from build123d import *

# Parameters (mm, degrees)
PRISM070_DEPTH                = 10
PRISM070_PITCH_ANGLE          = 90
PRISM071_DEPTH                = 10
PRISM071_PITCH_ANGLE          = 90
PRISM072_DEPTH                = 10
PRISM072_PITCH_ANGLE          = 90
PRISM073_DEPTH                = 10
PRISM073_PITCH_ANGLE          = 90
CUBE082_W                     = 5
CUBE082_H                     = 35
CUBE082_DEPTH                 = 32
CUBE081_W                     = 16
CUBE081_H                     = 15.2
CUBE081_DEPTH                 = 30
CUBE077_W                     = 3
CUBE077_H                     = 11.7
CUBE077_DEPTH                 = 30
CUBE078_W                     = 3
CUBE078_H                     = 11.7
CUBE078_DEPTH                 = 30
CUBE079_W                     = 1.6
CUBE079_H                     = 1.6
CUBE079_DEPTH                 = 30
CUBE080_W                     = 1.6
CUBE080_H                     = 1.6
CUBE080_DEPTH                 = 30
CYLINDER021_R                 = 7.6
CYLINDER021_DEPTH             = 30
CYLINDER020_R                 = 9.2
CYLINDER020_DEPTH             = 30
DIFFERENCE050_ROLL_ANGLE      = 90
DIFFERENCE050_PLACEMENT_ANGLE = 90


with BuildPart() as prism070:
    # prism070 → prism070 (new body)
    with BuildSketch(Plane.XY):
        Polygon((1.6, 0), (1.52169, 0.494427), (1.294427, 0.940456), (0.940456, 1.294427), (0.494427, 1.52169), (0, 1.6), (-0.494427, 1.52169), (-0.940456, 1.294427), (-1.294427, 0.940456), (-1.52169, 0.494427), (-1.6, 0), (-1.52169, -0.494427), (-1.294427, -0.940456), (-0.940456, -1.294427), (-0.494427, -1.52169), (0, -1.6), (0.494427, -1.52169), (0.940456, -1.294427), (1.294427, -0.940456), (1.52169, -0.494427), align=None)
    extrude(amount=PRISM070_DEPTH)


with BuildPart() as prism070_1:
    # prism070 pitch: moved
    add(prism070.part.rotate(Axis((0, 0, 0), (0, 1, 0)), PRISM070_PITCH_ANGLE))


with BuildPart() as prism070_2:
    # prism070 placement: moved
    add(prism070_1.part.moved(Location((-10, 12, 10))))


with BuildPart() as prism071:
    # prism071 → prism071 (new body)
    with BuildSketch(Plane.XY):
        Polygon((1.6, 0), (1.52169, 0.494427), (1.294427, 0.940456), (0.940456, 1.294427), (0.494427, 1.52169), (0, 1.6), (-0.494427, 1.52169), (-0.940456, 1.294427), (-1.294427, 0.940456), (-1.52169, 0.494427), (-1.6, 0), (-1.52169, -0.494427), (-1.294427, -0.940456), (-0.940456, -1.294427), (-0.494427, -1.52169), (0, -1.6), (0.494427, -1.52169), (0.940456, -1.294427), (1.294427, -0.940456), (1.52169, -0.494427), align=None)
    extrude(amount=PRISM071_DEPTH)


with BuildPart() as prism071_1:
    # prism071 pitch: moved
    add(prism071.part.rotate(Axis((0, 0, 0), (0, 1, 0)), PRISM071_PITCH_ANGLE))


with BuildPart() as prism071_2:
    # prism071 placement: moved
    add(prism071_1.part.moved(Location((-10, 12, -10))))


with BuildPart() as prism072:
    # prism072 → prism072 (new body)
    with BuildSketch(Plane.XY):
        Polygon((1.6, 0), (1.52169, 0.494427), (1.294427, 0.940456), (0.940456, 1.294427), (0.494427, 1.52169), (0, 1.6), (-0.494427, 1.52169), (-0.940456, 1.294427), (-1.294427, 0.940456), (-1.52169, 0.494427), (-1.6, 0), (-1.52169, -0.494427), (-1.294427, -0.940456), (-0.940456, -1.294427), (-0.494427, -1.52169), (0, -1.6), (0.494427, -1.52169), (0.940456, -1.294427), (1.294427, -0.940456), (1.52169, -0.494427), align=None)
    extrude(amount=PRISM072_DEPTH)


with BuildPart() as prism072_1:
    # prism072 pitch: moved
    add(prism072.part.rotate(Axis((0, 0, 0), (0, 1, 0)), PRISM072_PITCH_ANGLE))


with BuildPart() as prism072_2:
    # prism072 placement: moved
    add(prism072_1.part.moved(Location((-10, -12, 10))))


with BuildPart() as prism073:
    # prism073 → prism073 (new body)
    with BuildSketch(Plane.XY):
        Polygon((1.6, 0), (1.52169, 0.494427), (1.294427, 0.940456), (0.940456, 1.294427), (0.494427, 1.52169), (0, 1.6), (-0.494427, 1.52169), (-0.940456, 1.294427), (-1.294427, 0.940456), (-1.52169, 0.494427), (-1.6, 0), (-1.52169, -0.494427), (-1.294427, -0.940456), (-0.940456, -1.294427), (-0.494427, -1.52169), (0, -1.6), (0.494427, -1.52169), (0.940456, -1.294427), (1.294427, -0.940456), (1.52169, -0.494427), align=None)
    extrude(amount=PRISM073_DEPTH)


with BuildPart() as prism073_1:
    # prism073 pitch: moved
    add(prism073.part.rotate(Axis((0, 0, 0), (0, 1, 0)), PRISM073_PITCH_ANGLE))


with BuildPart() as prism073_2:
    # prism073 placement: moved
    add(prism073_1.part.moved(Location((-10, -12, -10))))


with BuildPart() as cube082:
    # cube082 → cube082 (new body)
    with BuildSketch(Plane(origin=(-9.5, -17.5, -16), x_dir=(1, 0, 0), z_dir=(0, 0, 1))):
        with Locations((2.5, 17.5)):
            Rectangle(CUBE082_W, CUBE082_H)
    extrude(amount=CUBE082_DEPTH)


with BuildPart() as union038:
    # cube081 → cube081 (new body)
    with BuildSketch(Plane(origin=(-16, -7.6, -15), x_dir=(1, 0, 0), z_dir=(0, 0, 1))):
        with Locations((8, 7.6)):
            Rectangle(CUBE081_W, CUBE081_H)
    extrude(amount=CUBE081_DEPTH)

    # union038: union prism070, prism071, prism072, prism073, cube082
    add(prism070_2.part)
    add(prism071_2.part)
    add(prism072_2.part)
    add(prism073_2.part)
    add(cube082.part)


with BuildPart() as cube077:
    # cube077 → cube077 (new body)
    with BuildSketch(Plane(origin=(-4.5, 4.95, -15), x_dir=(1, 0, 0), z_dir=(0, 0, 1))):
        with Locations((1.5, 5.85)):
            Rectangle(CUBE077_W, CUBE077_H)
    extrude(amount=CUBE077_DEPTH)


with BuildPart() as cube078:
    # cube078 → cube078 (new body)
    with BuildSketch(Plane(origin=(-4.5, -16.65, -15), x_dir=(1, 0, 0), z_dir=(0, 0, 1))):
        with Locations((1.5, 5.85)):
            Rectangle(CUBE078_W, CUBE078_H)
    extrude(amount=CUBE078_DEPTH)


with BuildPart() as cube079:
    # cube079 → cube079 (new body)
    with BuildSketch(Plane(origin=(-4.6, 7.5, -15), x_dir=(1, 0, 0), z_dir=(0, 0, 1))):
        with Locations((0.8, 0.8)):
            Rectangle(CUBE079_W, CUBE079_H)
    extrude(amount=CUBE079_DEPTH)


with BuildPart() as cube080:
    # cube080 → cube080 (new body)
    with BuildSketch(Plane(origin=(-4.6, -9.1, -15), x_dir=(1, 0, 0), z_dir=(0, 0, 1))):
        with Locations((0.8, 0.8)):
            Rectangle(CUBE080_W, CUBE080_H)
    extrude(amount=CUBE080_DEPTH)


with BuildPart() as cylinder021:
    # cylinder021 → cylinder021 (new body)
    with BuildSketch(Plane.XY.offset(-15)):
        Circle(CYLINDER021_R)
    extrude(amount=CYLINDER021_DEPTH)


with BuildPart() as difference050:
    # cylinder020 → cylinder020 (new body)
    with BuildSketch(Plane.XY.offset(-15)):
        Circle(CYLINDER020_R)
    extrude(amount=CYLINDER020_DEPTH)

    # difference049: cut cylinder021
    add(cylinder021.part, mode=Mode.SUBTRACT)

    # union037: union cube077, cube078, cube079, cube080
    add(cube077.part)
    add(cube078.part)
    add(cube079.part)
    add(cube080.part)

    # difference050: cut union038
    add(union038.part, mode=Mode.SUBTRACT)


with BuildPart() as difference050_1:
    # difference050 roll: moved
    add(difference050.part.rotate(Axis((0, 0, 0), (1, 0, 0)), DIFFERENCE050_ROLL_ANGLE))


with BuildPart() as difference050_2:
    # difference050 placement: moved
    add(difference050_1.part.moved(Location((298, 252, 340))).rotate(Axis((298, 252, 340), (0, 0, 1)), DIFFERENCE050_PLACEMENT_ANGLE))


solid = difference050_2.part
Source: CAD feature listing. Evaluate the final solid. Frame: model axes, mm. A direction names the side the tool comes from. Give positions to 0.01 mm unless a question says otherwise; leave off trailing zeros. Write each loop counter-clockwise with the first axis right and the second up, starting at its lowest first coordinate (ties: lowest second). Pieces come first, ordered by that corner, then holes. Notation, with made-up numbers: M -22.75,10.5 L -8.75,10.5 A36 ccw -8.75,49.5 Z; hole C -8.5,-27.5 d5. An arc over 180 degrees is marked long. Return JSON: item names as keys, results as strings. Group by question number.
1) Cut plane D-D, the plane z = 340. Output: boundary loops of the cut face in (x, y).
2) Cut plane A-A, the plane y = 249.25. Give the number of separate pieces and of enclosed holes in the cut face, plus the area to 3 significant figures.
3) Pull-direction query (Z, two-part tool) for faces 1 (the face through (298, 250.5, 327)), 2 (the face through (297.79, 259.6, 339.83)), 3 (the face through (297.79, 261.197, 339.777)); classes: pulls with the +Z half, pulls with the -Z half, needs draft (parallel to the pull), parting line crosses it, or undercut.
4) Material intervals for line 1 along Z through (x, y) = (310, 252.25); line 2 along Z through (x, y) = (295.5, 248.75); line 3 along Y through (x, z) = (310.5, 328), sorted ascending. Write a range as [from, to].
5) Set-up query: faces 4 (the face through (298, 247.5, 352)), 5 (the face through (298, 250, 347.6)). Return all of +Z, -Z, +X, -X, +Y, -Y with unobstructed straight access to the full face (end or side cutting, diameter ignored); none if empty.
6) Pin query (flat end, axial travel): P1, Ø4, axis at x = 300.5, z = 326, coming from the +Y side; P2, Ø1.5, axis at x = 290.5, z = 345, coming from the -Y side; P3, Ø8, axis at x = 288, z = 342, coming from the -Y side; P4, Ø3.5, axis at x = 293, y = 251, coming from the -Z side. Return the tip coordinate at first contact, or that it passes through.
7) Cut plane C-C, the plane x = 303.75. Output: boundary loops of the cut face in (y, z), plus the area to 3 significant figures.
8) Cut plane B-B, the plane y = 255.25. Output: boundary loops of the cut face in (x, z).
Recorded:
{
 "1": {"outline": "M 283,259.6 L 313,259.6 L 313,261.2 L 283,261.2 Z"},
 "2": {"separate pieces": "2", "enclosed holes": "4", "area": "511 mm²"},
 "3": {"face 1": "needs draft", "face 2": "undercut", "face 3": "parting line crosses it"},
 "4": {"line 1": "z = [330.8, 332.4], [347.6, 349.2]", "line 2": "z = [323.35, 332.4], [347.6, 356.65]", "line 3": "y = [247.5, 250.5]"},
 "5": {"face 4": "+Z, -Z, +X, -X, -Y", "face 5": "+X, -X, -Y"},
 "6": {"P1": "stops at y = 250.5", "P2": "stops at y = 256.97", "P3": "stops at y = 256.66", "P4": "stops at z = 323.35"},
 "7": {"outline": "M 247.5,323.35 L 250.5,323.35 L 250.5,330.92 A9.2 ccw long 250.5,349.08 L 250.5,356.65 L 247.5,356.65 L 247.5,347.6 L 252,347.6 A7.6 cw 252,332.4 L 247.5,332.4 Z", "area": "101 mm²"},
 "8": {"outline": "M 283,331.39 L 313,331.39 L 313,333.13 L 283,333.13 Z; M 283,346.87 L 313,346.87 L 313,348.61 L 283,348.61 Z"}
}
